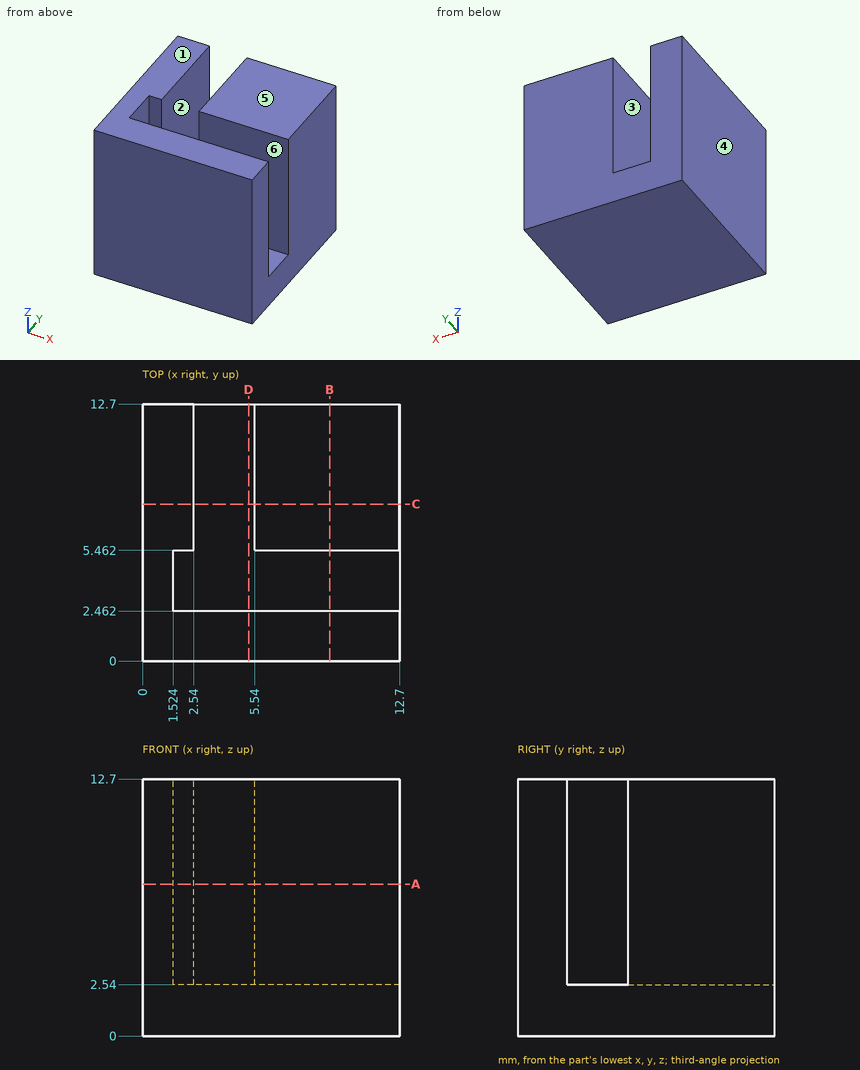
Here's the drawing with two shaded views (mm, measured from the low corner). I have some questions. A direction names the side the tool comes from. Give positions to 0.01 mm unless a question says otherwise; leave off trailing zeros. Order: outer loops, then holes, each group sorted by start corner. A loop starts at its lowest first (then second) coordinate and runs counter-clockwise, first axis right, second up. Notation, with made-up numbers: (71.5, 82.5) -> (98.5, 82.5) arc R32 ccw to (98.5, 112.5) -> close; hole circle Ø2 at (-25, -30.75). An arc over 180 degrees is marked (long way). One line per item, written item: value. Start each with the question number.
1. For the marked faces 5 and 6, which set-ups out of +Z, -Z, +X, -X, +Y, -Y let a thin tool reach every point of the face, with its end or its side?
2. I need wall thicknesses on probe 1 along Y at (x, z) = (2, 7.75); probe 2 along X at (y, z) = (12.25, 11); probe 3 along Z at (x, y) = (7.25, 3.75). Which ranges of each line are inside material? Lowest first, please. Write a range as from..to.
3. Imagine slicing it at A-A, the plane z = 7.5. List the corners of the cut face in (x, y) for me, plus the area to 3 significant figures.
4. Will this pin go through, and if not, where does the flat tip stop? pin 1 Ø0.9 at (y, z) = (4.5, 8) entering from +X.
5. Imagine slicing it at D-D, the plane x = 5.25. List the corners of the cut face in (y, z) for me.
6. Imagine slicing it at B-B, the plane x = 9.25. List the corners of the cut face in (y, z) for me.
7. We'd pull the mould along X, two halves only. Please class the marked faces 1, 2, 3 and 4: released by +X, released by -X, zero draft, split by the parting line, or undercut.
8. Imagine slicing it at C-C, the plane y = 7.75. List the corners of the cut face in (x, z) for me, plus the area to 3 significant figures.
Values follow:
1. face 5: +Z, +X, -X, +Y, -Y
1. face 6: +Z, +X
2. probe 1: y = 0..2.46, 5.46..12.7
2. probe 2: x = 0..2.54, 5.54..12.7
2. probe 3: z = 0..2.54
3. outline: (0, 0) -> (12.7, 0) -> (12.7, 2.46) -> (1.52, 2.46) -> (1.52, 5.46) -> (2.54, 5.46) -> (2.54, 12.7) -> (0, 12.7) -> close; (5.54, 5.46) -> (12.7, 5.46) -> (12.7, 12.7) -> (5.54, 12.7) -> close
3. area: 106 mm2
4. pin 1: stops at x = 1.52
5. outline: (0, 0) -> (12.7, 0) -> (12.7, 2.54) -> (2.46, 2.54) -> (2.46, 12.7) -> (0, 12.7) -> close
6. outline: (0, 0) -> (12.7, 0) -> (12.7, 12.7) -> (5.46, 12.7) -> (5.46, 2.54) -> (2.46, 2.54) -> (2.46, 12.7) -> (0, 12.7) -> close
7. face 1: zero draft
7. face 2: undercut
7. face 3: undercut
7. face 4: released by -X
8. outline: (0, 0) -> (12.7, 0) -> (12.7, 12.7) -> (5.54, 12.7) -> (5.54, 2.54) -> (2.54, 2.54) -> (2.54, 12.7) -> (0, 12.7) -> close
8. area: 131 mm2
